Autodesk Inventor part; units mm, degrees
ref_plane "YZ Plane" through (0, 0, 0) normal (1, 0, 0) x (0, 1, 0)
ref_plane "XZ Plane" through (0, 0, 0) normal (0, 1, 0) x (-1, 0, 0)
ref_plane "XY Plane" through (0, 0, 0) normal (0, 0, 1) x (1, 0, 0)
sketch "Skizze1" plane through (0, 0, 0) normal (0, 0, 1) x (1, 0, 0)
  line L0 (18, 18) -> (18, 0) construction
  line L1 (2, 18) -> (18, 18) construction
  line L2 (2, 0) -> (2, 18) construction
  line L3 (18, 0) -> (2, 0) construction
  line L4 (2, 18) -> (18, 18)
  line L5 (18, 0) -> (2, 0)
  line L6 (0.5764, 6.9713) -> (-2.7403, -18.928) construction
  circle A0 centre (14.2155, 15.0333) radius 1.2952 construction
  circle A1 centre (14.2155, 5.2246) radius 1.25 construction
  line L7 (2, 18) -> (-5.9127, 18)
  line L8 (-5.9127, 18) -> (-5.9127, 0)
  line L9 (-5.9127, 0) -> (2, 0)
  line L10 (18, 15.0333) -> (3.145, 15.0333) construction
  line L11 (18, 16.6333) -> (3.145, 16.6333)
  line L12 (3.145, 13.4333) -> (18, 13.4333)
  arc A2 (3.145, 16.6333) -> (3.145, 13.4333) centre (3.145, 15.0333) ccw
  line L13 (18, 5.2246) -> (3.145, 5.2246) construction
  line L14 (18, 6.8246) -> (3.145, 6.8246)
  line L15 (3.145, 3.6246) -> (18, 3.6246)
  arc A3 (3.145, 6.8246) -> (3.145, 3.6246) centre (3.145, 5.2246) ccw
  line L16 (-5.9127, 18) -> (18, 18)
  line L17 (18, 0) -> (-5.9127, 0)
  line L18 (-5.9127, 0) -> (-5.9127, 18)
  line L19 (18, 16.6333) -> (3.145, 16.6333)
  line L20 (18, 13.4333) -> (3.145, 13.4333)
  line L21 (18, 6.8246) -> (3.145, 6.8246)
  line L22 (18, 3.6246) -> (3.145, 3.6246)
  line L23 (18, 18) -> (18, 16.6333)
  line L24 (18, 18) -> (18, 16.6333)
  line L25 (18, 13.4333) -> (18, 6.8246)
  line L26 (18, 3.6246) -> (18, 0)
  line L27 (18, 13.4333) -> (18, 6.8246)
  line L28 (18, 3.6246) -> (18, 0)
  point P0 (0, 0)
  point P1 (10.5725, 15.0333)
  point P2 (10.5725, 5.2246)
  dimension "d0" = 2.5
  dimension "d1" = 3.2
  dimension "d2" = 3.2
extrude "Extrusion1" add sketch "Skizze1" along normal blind 10
sketch "Skizze2" plane through (0, 0, 10) normal (0, 0, 1) x (1, 0, 0)
  line L0 (-5.9127, 0) -> (18, 0) construction
  line L1 (18, 0) -> (18, 3.6246) construction
  line L2 (18, 3.6246) -> (3.145, 3.6246) construction
  arc A0 (3.145, 6.8246) -> (3.145, 3.6246) centre (3.145, 5.2246) ccw construction
  line L3 (3.145, 6.8246) -> (18, 6.8246) construction
  line L4 (18, 6.8246) -> (18, 13.4333) construction
  line L5 (18, 13.4333) -> (3.145, 13.4333) construction
  arc A1 (3.145, 16.6333) -> (3.145, 13.4333) centre (3.145, 15.0333) ccw construction
  line L6 (3.145, 16.6333) -> (18, 16.6333) construction
  line L7 (18, 16.6333) -> (18, 18) construction
  line L8 (18, 18) -> (-5.9127, 18) construction
  line L9 (-5.9127, 18) -> (-5.9127, 0) construction
  line L10 (18, 18) -> (-5.9127, 18)
  line L11 (-5.9127, 0) -> (18, 0)
  line L12 (18, 18) -> (-3, 18)
  line L13 (-3, 18) -> (-3, 0)
  line L14 (-3, 0) -> (18, 0)
  line L15 (18, 0) -> (18, 18)
  point P0 (0, 0)
  dimension "d5" = 21
extrude "Extrusion2" cut sketch "Skizze2" against normal blind 8
fillet "Rundung1" radius 1 7 edges at (-5.9127, 18, 5) (-3, 18, 6) (-3, 9, 10) (-5.9127, 9, 10) (-4.4563, 0, 10) (7.5, 18, 2) (7.5, 0, 2)
properties part number "Pusher"
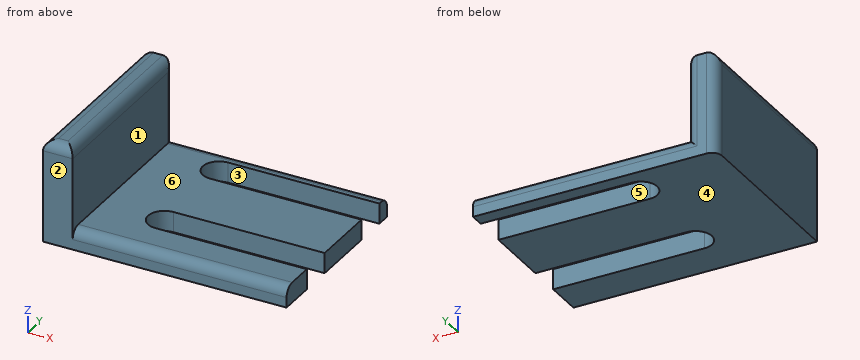
Geometry check sheet. Reference: the model listing, model coordinates, mm. Face numbers are marked on the shaded views. A direction names the side the tool comes from. Coordinates: 2 decimals unless noted, no trailing zeros. Order: outer loops, then holes, each group sorted by start corner. A loop starts at its lowest first (then second) coordinate and runs counter-clockwise, first axis right, second up. Notation, with made-up numbers: M -5,-39 L 30,-39 A20 cw 30,-13 Z; hole C 48.5,74.25 d8. An arc over 180 degrees is marked long. Answer as a JSON object with one key per item and string values.
Q1. Cross-section at D-D on x = 1. Record the cut outline in (y, z).
Results are:
{"outline": "M 0,0 L 18,0 L 18,1 A1 ccw 17,2 L 1,2 A1 ccw 0,1 Z"}
Q2. Scan lines: line 1 (Y direction, x = 4, z = 1); line 2 (X direction, y = 4.5, z = 6.5); line 3 (Z direction, x = 7.5, y = 9.75). Record each from-to range of solid material in increasing order.
Results are:
{"line 1": "y = 0 to 3.62, 6.82 to 13.43, 16.63 to 18", "line 2": "x = -5.91 to -3", "line 3": "z = 0 to 2"}
Q3. Tool access check on the marked faces 4, 5 and 6. Record the directions out of +Z, -Z, +X, -X, +Y, -Y that give a thin tool (end or side, any length) a straight path to the whole face; none if there is none.
Results are:
{"face 4": "-Z, +X, -X, +Y, -Y", "face 5": "+Z, -Z, +X", "face 6": "+Z, +X, +Y, -Y"}
Q4. Cross-section at B-B on y = 10. Record the cut outline in (x, z).
Results are:
{"outline": "M -5.91,0 L 18,0 L 18,2 L -3,2 L -3,9 A1 ccw -4,10 L -4.91,10 A1 ccw -5.91,9 Z"}
Q5. Cross-section at C-C on z = 8.5. Record the cut outline in (x, y).
Results are:
{"outline": "M -5.91,0 L -3,0 L -3,17 A1 ccw -4,18 L -4.91,18 A1 ccw -5.91,17 Z"}
Q6. Cross-section at A-A on x = 16. Record the cut outline in (y, z).
Results are:
{"outline": "M 0,0 L 3.62,0 L 3.62,2 L 1,2 A1 ccw 0,1 Z; M 6.82,0 L 13.43,0 L 13.43,2 L 6.82,2 Z; M 16.63,0 L 18,0 L 18,1 A1 ccw 17,2 L 16.63,2 Z"}
Q7. Release check for a two-part mould opening along Y. For the marked faces 1, 2 and 3 record: released by +Y, released by -Y, zero draft, split by the parting line, or undercut.
Results are:
{"face 1": "zero draft", "face 2": "released by -Y", "face 3": "undercut"}
Q8. Depth check by flat-ended pin: pin 1 Ø10 at (x, y) = (3, 15.5) entering from +Z; pin 2 Ø2 at (x, z) = (14.5, 2.5) entering from +Y. Enter the tip coordinate at first touch or a pass-through.
Results are:
{"pin 1": "stops at z = 2", "pin 2": "stops at y = 17.87"}
